The drawing under review shows one solid part. Ordinate dimensions are in mm from its lowest x, y, z. A direction names the side the tool comes from. Give positions to 0.01 mm unless a question says otherwise; leave off trailing zeros. Write each loop counter-clockwise with the first axis right and the second up, starting at its lowest first coordinate (ties: lowest second). Pieces come first, ordered by that corner, then holes.
Q1. Mouldability with a two-part tool opening along X and no side actions: class the marked faces 3, 4, 5 and 6 as released by +X, released by -X, zero draft, split by the parting line, or undercut.
Q2. Insertion check: P1, Ø6, axis at y = 88, z = 21, coming from the -X side; P2, Ø8, axis at x = 128.74, z = 25, coming from the +Y side; P3, Ø1, axis at x = 55.5, y = 130.5, coming from the -Z side; P4, Ø10, axis at x = 50, y = 153.5, coming from the -Z side. Each pin has a flat end and moves straight along its axis. Give the tip position at first contact, or say it passes through.
Q3. We need section B-B (z = 14.5). Write out the cut boundary in (x, y).
Q4. Machinability: for the marked faces 1 and 2, which of the approach directions +Z, -Z, +X, -X, +Y, -Y give a long, thin tool a straight path to every point of the face, cutting with its end or side? Answer none if there is none.
Q5. For line 1 (Y direction, x = 33.5, z = 5); line 2 (X direction, y = 25.5, z = 7.5), list the stretches that pass through material, from the lowest coordinate up.
Q6. We need section A-A (z = 25). Write out the cut boundary in (x, y).
Q7. We need section C-C (x = 17.5). Write out the cut boundary in (y, z), then the cut area to 3 significant figures.
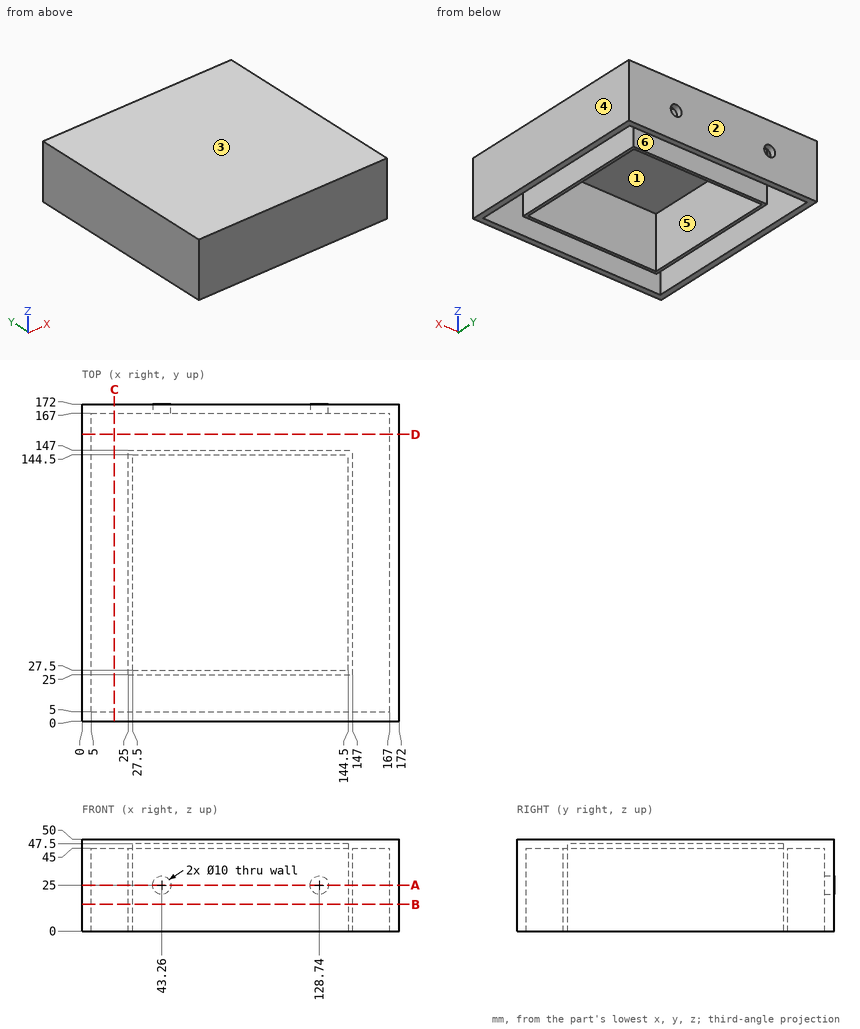
Computed:
1. face 3: zero draft
1. face 4: released by +X
1. face 5: undercut
1. face 6: undercut
2. P1: stops at x = 0
2. P2: stops at y = 147
2. P3: stops at z = 47.5
2. P4: stops at z = 45
3. outline: (0, 0) - (172, 0) - (172, 172) - (0, 172) - close; (25, 25) - (147, 25) - (147, 147) - (25, 147) - close; hole (5, 5) - (167, 5) - (167, 167) - (5, 167) - close; hole (27.5, 27.5) - (144.5, 27.5) - (144.5, 144.5) - (27.5, 144.5) - close
4. face 1: -Z
4. face 2: +Z, -Z, +X, -X, +Y
5. line 1: y = 0 to 5, 25 to 27.5, 144.5 to 147, 167 to 172
5. line 2: x = 0 to 5, 25 to 147, 167 to 172
6. outline: (0, 0) - (172, 0) - (172, 172) - (133.74, 172) - (133.74, 167) - (167, 167) - (167, 5) - (5, 5) - (5, 167) - (38.26, 167) - (38.26, 172) - (0, 172) - close; (25, 25) - (147, 25) - (147, 147) - (25, 147) - close; (48.26, 167) - (123.74, 167) - (123.74, 172) - (48.26, 172) - close; hole (27.5, 27.5) - (144.5, 27.5) - (144.5, 144.5) - (27.5, 144.5) - close
7. outline: (0, 0) - (5, 0) - (5, 45) - (167, 45) - (167, 0) - (172, 0) - (172, 50) - (0, 50) - close
7. area: 1,310 mm2
